```python
from build123d import *


with BuildPart() as part:
    # Sketch1 → Revolve2 (revolve)
    with BuildSketch(Plane.XY):
        with BuildLine():
            Line((-9, -7.5), (-9, 0))
            Line((-9, 0), (0, 0))
            Line((0, 0), (0, 2))
            Line((0, 2), (0, 14.5))
            ThreePointArc((0, 14.5), (-4.526641021, 11.623563296), (-3.845043489, 6.303808428))
            add(Edge.make_bspline(
                [(-6.655258628, 2), (-6.120506519, 2), (-5.250490252, 2.299992699), (-3.576908903, 3.35585887), (-2.957362509, 5.235921257), (-3.845043489, 6.303808428)],
                knots=[0, 0, 0, 0, 0.245004217, 0.484762515, 1, 1, 1, 1], degree=3))
            Line((-6.655258628, 2), (-8, 2))
            Line((-8, 2), (-9.37373871, 2.5))
            Line((-9.37373871, 2.5), (-11, 2.5))
            Line((-11, 2.5), (-11.5, 2))
            Line((-11.5, 2), (-11.5, 0.37373871))
            Line((-11.5, 0.37373871), (-11, -1))
            Line((-11, -1), (-11, -7.5))
            Line((-11, -7.5), (-9, -7.5))
        make_face()
    revolve(axis=Axis((0, 14.5, 0), (0, -1, 0)))


solid = part.part
```
Read the model definition and answer for the solid it produces. Units are mm, in the model's axes. A direction names the side the tool comes from. Coordinates: 2 decimals unless noted, no trailing zeros.
(1) Consider line 1 along Z through (x, y) = (0, -2); line 2 along Y through (x, z) = (-9.75, -3.25). Determine where each line is inside the solid, lowest interval first.
Solution:
line 1: z = -11 to -9, 9 to 11
line 2: y = -7.5 to 2.5
(2) The mould has two halves that part along X. Classify faces 3 (the face through (2.38, -4.3, 10.74)), 4 (the face through (-4.9, 2.5, -8.2)), 5 (the face through (0, 0, 0)), 6 (the face through (-7, 2, -1)): released by +X, released by -X, zero draft, split by the parting line, or undercut.
Solution:
face 3: split by the parting line
face 4: zero draft
face 5: undercut
face 6: undercut
(3) A tool of negligible diameter and unlimited length cuts with its end or side. For faces 1 (the face through (-2, -7.5, 9)), 2 (the face through (1.172, -3.698, -8.923)), from which of +Z, -Z, +X, -X, +Y, -Y can it reach the whole face along a straight path? Write none if from no direction.
Solution:
face 1: +Z, -Z, +X, -X, -Y
face 2: -Y
(4) Flat-ended cylindrical pins translate along their axes: pin 1 Ø1 at (x, y) = (6, 1.5) entering from +Z; pin 2 Ø1.5 at (x, y) = (1.5, 11.5) entering from +Z; pin 3 Ø3 at (x, y) = (-1, 11.5) entering from -Z. Find the tip coordinate at first contact, or state that the pin passes through.
Solution:
pin 1: stops at z = 10.1
pin 2: stops at z = 4.68
pin 3: stops at z = -4.95
